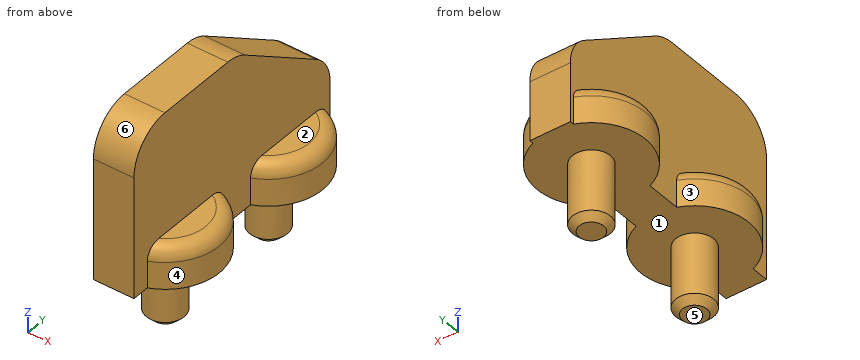
from build123d import *

# Parameters (mm, degrees)
F0_R     = 1.4
F1_DEPTH = 12
F2_DEPTH = 5
F3_SIZE  = 0.5
F4_DEPTH = 3
F5_R     = 1
F7_DEPTH = 25
F8_R     = 3


# Not quite as in the source:
# - a pattern or mirror of a feature is missing from the dataset's text; its kind, count and spacing are read off the source's solid
# - a feature names something its author has since deleted; it is built from what else it names


with BuildPart() as f1:
    # F0 (on Top) → F1 (new body)
    with BuildSketch(Plane.XY):
        with BuildLine():
            ThreePointArc((1.5, 8.7080992435), (0.7640690498, 8.92634671), (0, 9))
            ThreePointArc((0, 9), (-0.7640690498, 8.92634671), (-1.5, 8.7080992435))
            Line((-1.5, 8.7080992435), (-1.5, 1.2919007565))
            Line((-1.5, 1.2919007565), (-1.5, -1.2919007565))
            Line((-1.5, -1.2919007565), (-1.5, -8.7080992435))
            Line((-1.5, -8.7080992435), (-1.5, -10))
            Line((-1.5, -10), (1.5, -10))
            Line((1.5, -10), (1.5, -8.7080992435))
            Line((1.5, -8.7080992435), (1.5, -1.2919007565))
            Line((1.5, -1.2919007565), (1.5, 1.2919007565))
            Line((1.5, 1.2919007565), (1.5, 8.7080992435))
        make_face()
        with Locations((0, -5)):
            Circle(F0_R, mode=Mode.SUBTRACT)
        with Locations((0, 5)):
            Circle(F0_R, mode=Mode.SUBTRACT)
        with Locations((0, 5)):
            Circle(F0_R)
        with Locations((0, -5)):
            Circle(F0_R)
        with BuildLine():
            Line((0, 9), (-1.5, 9))
            Line((-1.5, 9), (-1.5, 8.7080992435))
            ThreePointArc((-1.5, 8.7080992435), (-0.7640690498, 8.92634671), (0, 9))
        make_face()
        with BuildLine():
            Line((1.5, 9), (0, 9))
            ThreePointArc((0, 9), (0.7640690498, 8.92634671), (1.5, 8.7080992435))
            Line((1.5, 8.7080992435), (1.5, 9))
        make_face()
    extrude(amount=F1_DEPTH)

    # F0 (on Top) → F2 (join)
    with BuildSketch(Plane.XY):
        with Locations((0, 5)):
            Circle(F0_R)
    f2 = extrude(amount=-F2_DEPTH)

    # F2_copies: F2 across plane
    add(f2.mirror(Plane(origin=(0, 0, 0), x_dir=(0, 0, -1), z_dir=(0, -1, 0))))

    # F3
    f3_edges = [f1.edges().sort_by_distance(p)[0] for p in [
        (-1.4, -5, -5),
        (-1.4, 5, -5),
    ]]
    chamfer(f3_edges, length=F3_SIZE)

    # F0 (on Top) → F4 (join)
    with BuildSketch(Plane.XY):
        with Locations((0, 5)):
            Circle(F0_R)
        with Locations((0, -5)):
            Circle(F0_R)
        with BuildLine():
            Line((0, 9), (-1.5, 9))
            Line((-1.5, 9), (-1.5, 8.7080992435))
            ThreePointArc((-1.5, 8.7080992435), (-0.7640690498, 8.92634671), (0, 9))
        make_face()
        with BuildLine():
            Line((1.5, 9), (0, 9))
            ThreePointArc((0, 9), (0.7640690498, 8.92634671), (1.5, 8.7080992435))
            Line((1.5, 8.7080992435), (1.5, 9))
        make_face()
        with BuildLine():
            Line((-1.5, 1.2919007565), (-1.5, 8.7080992435))
            ThreePointArc((-1.5, 8.7080992435), (-4, 5), (-1.5, 1.2919007565))
        make_face()
        with BuildLine():
            ThreePointArc((1.5, 1.2919007565), (4, 5), (1.5, 8.7080992435))
            Line((1.5, 8.7080992435), (1.5, 1.2919007565))
        make_face()
        with BuildLine():
            Line((-1.5, -8.7080992435), (-1.5, -1.2919007565))
            ThreePointArc((-1.5, -1.2919007565), (-4, -5), (-1.5, -8.7080992435))
        make_face()
        with BuildLine():
            ThreePointArc((1.5, -8.7080992435), (4, -5), (1.5, -1.2919007565))
            Line((1.5, -1.2919007565), (1.5, -8.7080992435))
        make_face()
    extrude(amount=F4_DEPTH)

    # F5
    f5_edges = [f1.edges().sort_by_distance(p)[0] for p in [
        (-4, -5, 3),
        (4, -5, 3),
        (-4, 5, 3),
        (4, 5, 3),
    ]]
    fillet(f5_edges, radius=F5_R)

    # F6 (on face) → F7 (cut)
    with BuildSketch(Plane(origin=(-1.5, 0, 0), x_dir=(0, -1, 0), z_dir=(-1, 0, 0))):
        Polygon((0, 12), (-9, 12), (-9, 6), align=None)
    extrude(amount=-F7_DEPTH, mode=Mode.SUBTRACT)

    # F8
    f8_edges = [f1.edges().sort_by_distance(p)[0] for p in [
        (0, -10, 12),
        (0, 0, 12),
        (0, 9, 6),
    ]]
    fillet(f8_edges, radius=F8_R)


solid = f1.part
Work out the finished part from the listing and answer in its coordinate system (mm). Face numbers are marked on the shaded views. A direction names the side the tool comes from. Round coordinates to 2 decimals unless told otherwise and drop trailing zeros. Order: outer loops, then holes, each group sorted by start corner. A loop starts at its lowest first (then second) coordinate and runs counter-clockwise, first axis right, second up. Notation, with made-up numbers: M 17.5,78.25 L 68.5,78.25 A22 cw 68.5,93.25 Z; hole C 29,47 d5. An arc over 180 degrees is marked long. Put each result on its own line as item: value. Start each with the question number.
Q1. Straight lines are drawn through the part: L1, parallel to Y at x = 0, z = -3.25; L2, parallel to X at y = 5, z = 7; L3, parallel to Z at x = 0, y = -1.75. For each, find the intervals that lie inside material, in ascending order. Write a range as [from, to].
Q2. Section A-A, the plane y = -5 is taken. Write down the section's boundary in (x, z).
Q3. Section D-D, the plane z = 6 is taken. Write down the section's boundary in (x, y).
Q4. Flat-ended cylindrical pins translate along their axes: pin 1 (3 mm diameter, centred on y = 7, z = -1, fed in from -X); pin 2 (4 mm diameter, centred on x = 0.5, y = -2, fed in from -Z); pin 3 (1.7 mm diameter, centred on x = 2, y = -4, fed in from +Z); pin 4 (1 mm diameter, centred on x = 2.5, y = 2.5, fed in from -Z). Find the tip coordinate at first contact, or state that the pin passes through.
Q5. Section C-C, the plane z = -0.5 is taken. Write down the section's boundary in (x, y).
Q6. A tool of negligible diameter and unlimited length cuts with its end or side. For the marked faces 1, 2 and 3, from which of +Z, -Z, +X, -X, +Y, -Y can it reach the whole face along a straight path? Write none if from no direction.
Q7. Section B-B, the plane x = 0 is taken. Write down the section's boundary in (y, z).
Q8. For a pull along Y with two mould halves and no side action, classify the marked faces 4, 5 and 6 as pulls with the +Y half, pulls with the -Y half, needs draft (parallel to the pull), parting line crosses it, or undercut.
Findings below:
1. L1: y = [-6.4, -3.6], [3.6, 6.4]
1. L2: x = [-1.5, 1.5]
1. L3: z = [0, 12]
2. outline: M -4,0 L -1.4,0 L -1.4,-4.5 L -0.9,-5 L 0.9,-5 L 1.4,-4.5 L 1.4,0 L 4,0 L 4,2 A1 ccw 3,3 L 1.5,3 L 1.5,12 L -1.5,12 L -1.5,3 L -3,3 A1 ccw -4,2 Z
3. outline: M -1.5,-10 L 1.5,-10 L 1.5,8.53 L -1.5,8.53 Z
4. pin 1: stops at x = -3.9
4. pin 2: stops at z = -4.86
4. pin 3: stops at z = 12
4. pin 4: stops at z = 0
5. outline: C 0,-5 d2.8; C 0,5 d2.8
6. face 1: -Z
6. face 2: +Z, +X, +Y, -Y
6. face 3: +Z, -Z, -X
7. outline: M -10,0 L -6.4,0 L -6.4,-4.5 L -5.9,-5 L -4.1,-5 L -3.6,-4.5 L -3.6,0 L 3.6,0 L 3.6,-4.5 L 4.1,-5 L 5.9,-5 L 6.4,-4.5 L 6.4,0 L 9,0 L 9,4.39 A3 ccw 7.66,6.89 L 0.76,11.5 A3 ccw -0.91,12 L -7,12 A3 ccw -10,9 Z
8. face 4: undercut
8. face 5: needs draft
8. face 6: pulls with the -Y half
